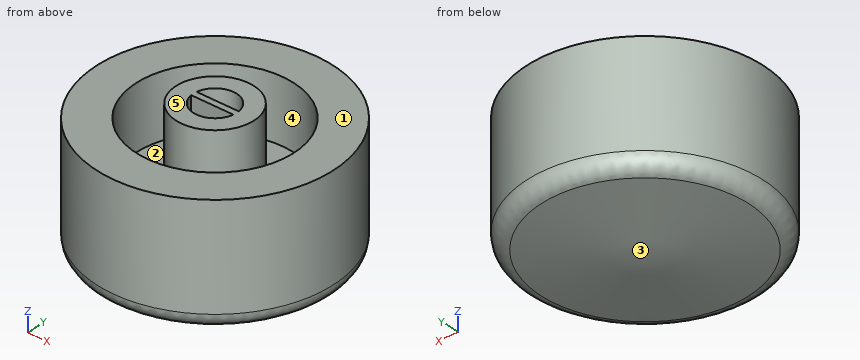
```python
from build123d import *

# Parameters (mm, degrees)
FILLET1_R           = 2
SKETCH5_W           = 5.905041088
SKETCH5_H           = 0.8
BOSS_EXTRUDE4_DEPTH = 13


with BuildPart() as part:
    # Sketch1 → Revolve1 (revolve)
    with BuildSketch(Plane(origin=(0, 0, 0), x_dir=(1, 0, 0), z_dir=(0, 1, 0))):
        Polygon((2.75, 40.602114639), (2.75, 53.602114639), (0, 53.602114639), (0, 58.602114639), (15, 57.289784686), (15, 42.289784686), (10, 42.289784686), (10, 50.278222223), (4.95, 50.278222223), (4.95, 40.602114639), align=None)
    revolve(axis=Axis((0, 0, -53.602114639), (0, 0, -1)))

    # Fillet1
    fillet1_edges = [part.edges().sort_by_distance(p)[0] for p in [
        (-15, 0, -57.289784686),
    ]]
    fillet(fillet1_edges, radius=FILLET1_R)

    # Sketch5 → Boss-Extrude4 (add)
    with BuildSketch(Plane.XY.offset(-53.602114639)):
        with Locations((-0.048658074, 0)):
            Rectangle(SKETCH5_W, SKETCH5_H)
    extrude(amount=BOSS_EXTRUDE4_DEPTH)


solid = part.part
```
Source: CAD feature listing. Evaluate the final solid. Frame: model axes, mm. Face numbers are marked on the shaded views. A direction names the side the tool comes from. Coordinates: 2 decimals unless noted, no trailing zeros. Loops run counter-clockwise (first coordinate to the right, second up) from the corner with the lowest first, then second, coordinate; pieces in that order, holes last. Notation, with made-up numbers: M -17.5,75.25 L 4.5,75.25 A33 ccw 4.5,105.25 Z; hole C -5.5,-36.5 d8. An arc over 180 degrees is marked long. Put each result on its own line as item: value. Start each with the question number.
1) Contact query for flat-ended pins moving along their axis: pin 1 Ø10 at (x, z) = (9, -48) entering from -Y; pin 2 Ø2 at (x, y) = (6.5, -4) entering from -Z; pin 3 Ø12 at (x, y) = (-10.5, -11.5) entering from +Z. Output: stop coordinate, or through.
2) Pull-direction query (Y, two-part tool) for the marked faces 1, 2 and 3; classes: pulls with the +Y half, pulls with the -Y half, needs draft (parallel to the pull), parting line crosses it, or undercut.
3) Cut plane A-A on z = -48.5. Return the cut outline in (x, y), then the cut area to 3 significant figures.
4) Reachability of the marked faces 4 and 5 from +Z, -Z, +X, -X, +Y, -Y: full face, straight path, thin tool, end or side. Return the list, or none.
5) Ray query, L1, parallel to X at y = 0, z = -48.5; L2, parallel to Y at x = 0, z = -47.5; L3, parallel to Y at x = 4, z = -45.5. Return the intervals inside material, ascending. Write a range as from..to.
The answers:
1. pin 1: stops at y = -14.46
1. pin 2: stops at z = -58.02
1. pin 3: stops at z = -42.29
2. face 1: needs draft
2. face 2: undercut
2. face 3: parting line crosses it
3. outline: C 0,0 d30; C 0,0 d9.9; hole C 0,0 d20; hole M -2.72,-0.4 A2.75 ccw 2.72,-0.4 Z; hole M -2.72,0.4 L 2.72,0.4 A2.75 ccw Z
3. area: 450 mm²
4. face 4: +Z
4. face 5: +Z, +X, -X, +Y, -Y
5. L1: x = -15..-10, -4.95..4.95, 10..15
5. L2: y = -15..-10, -4.95..-2.75, -0.4..0.4, 2.75..4.95, 10..15
5. L3: y = -14.46..-9.17, -2.92..2.92, 9.17..14.46
